Could you check a few things on this model? Use its own coordinates, in mm. A direction names the side the tool comes from. Give positions to 0.01 mm unless a question says otherwise; leave off trailing zeros. Loops run counter-clockwise (first coordinate to the right, second up) from the corner with the lowest first, then second, coordinate; pieces in that order, holes last. Notation, with made-up numbers: (-3, 33.5) -> (36, 33.5) arc R9 cw to (36, 39.5) -> close; hole circle Ø9 at (-29, -27). An arc over 180 degrees is marked (long way). Put each result on its own line as item: value.
```python
from build123d import *

# Parameters (mm, degrees)
F1_DEPTH = 6
F2_R     = 2.99999
F3_R     = 1.5
F4_DEPTH = 39.751
F5_SIZE  = 2.5


# Not quite as in the source:
# - a fillet or chamfer is up to 0.001 mm smaller than in the source, because OpenCascade refuses the exact size


with BuildPart() as f1:
    # F0 (on Top) → F1 (new body)
    with BuildSketch(Plane.XY):
        Polygon((0, -5.7625164015), (0, -17.7625164015), (50, -17.7625164015), (50, -5.7625164015), (39.75, -5.7625164015), (39.75, 2.2374835985), (10.25, 2.2374835985), (10.25, -5.7625164015), align=None)
    extrude(amount=F1_DEPTH)

    # F2 (radius 3 in the source; OpenCascade refuses exactly that, so slightly less here)
    f2_edges = [f1.edges().sort_by_distance(p)[0] for p in [
        (25, 2.237484, 6),
        (25, 2.237484, 0),
        (5.125, -5.762516, 6),
        (44.875, -5.762516, 6),
        (5.125, -5.762516, 0),
        (44.875, -5.762516, 0),
    ]]
    fillet(f2_edges, radius=F2_R)

    # F3 (on face) → F4 (cut, through all)
    with BuildSketch(Plane(origin=(10.25, 0, 0), x_dir=(0, -1, 0), z_dir=(-1, 0, 0))):
        with Locations((1.5625164015, 3)):
            Circle(F3_R)
    extrude(amount=-F4_DEPTH, mode=Mode.SUBTRACT)

    # F5
    f5_edges = [f1.edges().sort_by_distance(p)[0] for p in [
        (25, -17.762516, 6),
    ]]
    chamfer(f5_edges, length=F5_SIZE)


solid = f1.part
```
1. If we section it at D-D (z = 0.5): List the corners of the cut face in (x, y) for me.
Recorded:
outline: (0, -17.76) -> (50, -17.76) -> (50, -7.1) -> (39.75, -7.1) -> (39.75, 0.9) -> (10.25, 0.9) -> (10.25, -7.1) -> (0, -7.1) -> close
2. If we section it at C-C (z = 3.95): List the corners of the cut face in (x, y) for me, then the cut area to 3 significant figures.
Recorded:
outline: (0, -17.31) -> (50, -17.31) -> (50, -5.92) -> (39.75, -5.92) -> (39.75, -2.72) -> (10.25, -2.72) -> (10.25, -5.92) -> (0, -5.92) -> close; (10.25, -0.4) -> (39.75, -0.4) -> (39.75, 2.08) -> (10.25, 2.08) -> close
area: 737 mm^2
3. Thinking about a two-plate mould opening in Z: for faces 5 (the face through (24.79, 1.38, 0.9)), 6 (the face through (44.8, -6.62, 5.1)), 7 (the face through (24.794, -1.237, 1.536)), 8 (the face through (0, -12, 3)), which applies, pulls with the +Z half, pulls with the -Z half, needs draft (parallel to the pull), parting line crosses it, or undercut?
Recorded:
face 5: pulls with the -Z half
face 6: pulls with the +Z half
face 7: undercut
face 8: needs draft
4. For faces 1 (the face through (5.05, -6.62, 5.1)), 2 (the face through (24.65, -16.53, 4.73)), 3 (the face through (5.05, -6.62, 0.9)), 4 (the face through (44.8, -6.62, 0.9)), which set-ups out of +Z, -Z, +X, -X, +Y, -Y let a thin tool reach every point of the face, with its end or its side?
Recorded:
face 1: +Z, -X, +Y
face 2: +Z, +X, -X, -Y
face 3: -Z, -X, +Y
face 4: -Z, +X, +Y
5. I need wall thicknesses on line 1 (Z direction, x = 28.5, y = -1.5); line 2 (X direction, y = -3.5, z = 5.25); line 3 (Y direction, x = 13, z = 2.7). Which ranges of each line are inside material? Lowest first, please.
Recorded:
line 1: z = 0 to 1.5, 4.5 to 6
line 2: x = 10.25 to 39.75
line 3: y = -17.76 to -3.03, -0.09 to 2.22
6. I'm going to push flat-ended pins straight in: pin 1 (1.5 mm diameter, centred on x = 31, z = 4.5, fed in from -Y); pin 2 (3 mm diameter, centred on y = -3.5, z = 4, fed in from +X); pin 3 (1.8 mm diameter, centred on y = -1.56, z = 3, fed in from +X). Where does each tip first touch, or does it pass through?
Recorded:
pin 1: stops at y = -17.51
pin 2: stops at x = 39.75
pin 3: passes through
